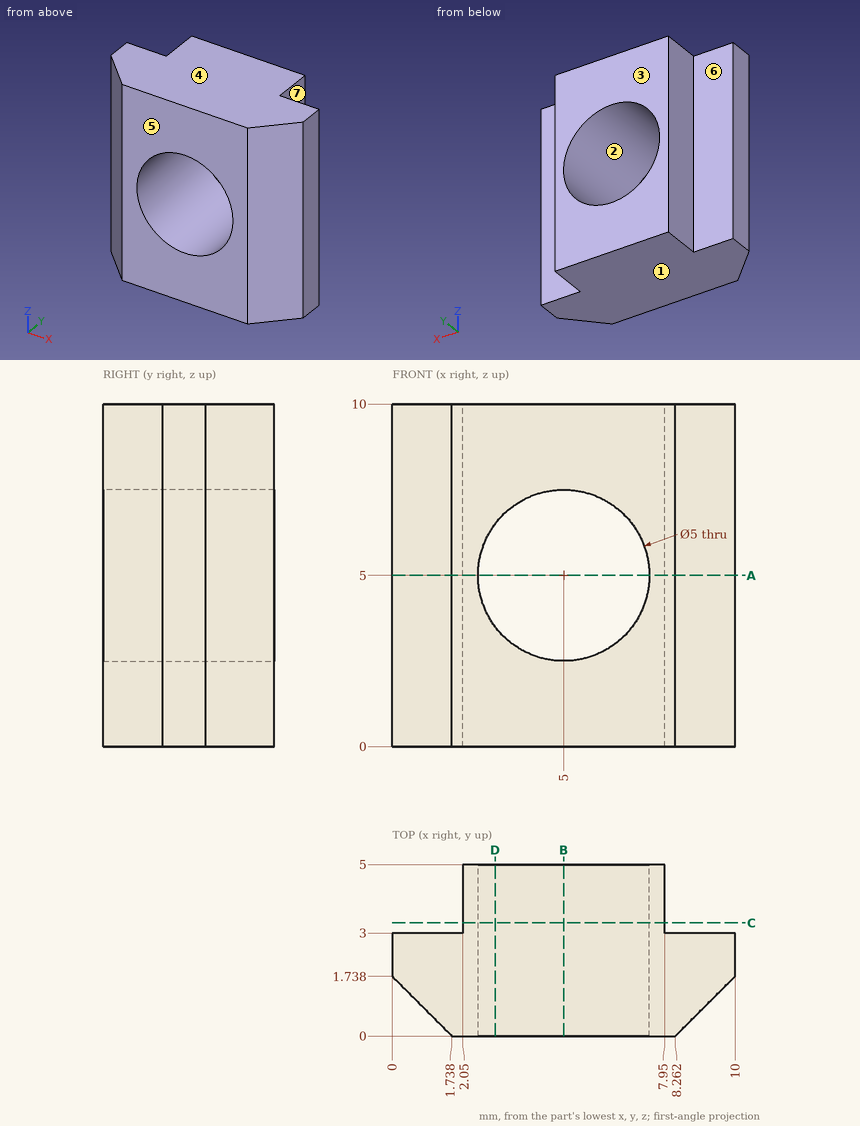
Study the drawing (mm; zero at the part's minimum x, y, z) and answer. A direction names the side the tool comes from. Round coordinates to 2 decimals unless told otherwise and drop trailing zeros. Loops run counter-clockwise (first coordinate to the right, second up) from the corner with the lowest first, then second, coordinate; pieces in that order, holes last.
Q1. Section A-A, the plane z = 5 is taken. Determine the outline of the cut face in (x, y).
Q2. Section B-B, the plane x = 5 is taken. Determine the outline of the cut face in (y, z).
Q3. Given pin 1 Ø1 at (x, z) = (9, 3) entering from +Y; pin 2 Ø1 at (y, z) = (4.5, 7) entering from +X; pin 3 Ø0.6 at (y, z) = (4, 6) entering from -X, each flat-ended and moving along its own axis, determine where each tip first touches the part or whether it passes through.
Q4. Section C-C, the plane y = 3.3 is taken. Determine the outline of the cut face in (x, z).
Q5. Find the intervals of material crossed by line 1 (X direction, y = 2.85, z = 5); line 2 (X direction, y = 4.45, z = 2); line 3 (X direction, y = 3.75, z = 5), in increasing order.
Q6. For a pull along Z with two mould halves and no side action, classify the marked faces 1, 2, 3 and 4 as released by +Z, released by -Z, zero draft, split by the parting line, or undercut.
Q7. Which of the six approach directions +Z, -Z, +X, -X, +Y, -Y give full straight-line access (tool end or side, diameter ignored) to the marked faces 5, 6 and 7?
Q8. Section D-D, the plane x = 3 is taken. Determine the outline of the cut face in (y, z).
Completed:
1. outline: (0, 1.74) - (1.74, 0) - (2.5, 0) - (2.5, 5) - (2.05, 5) - (2.05, 3) - (0, 3) - close; (7.5, 0) - (8.26, 0) - (10, 1.74) - (10, 3) - (7.95, 3) - (7.95, 5) - (7.5, 5) - close
2. outline: (0, 0) - (5, 0) - (5, 2.5) - (0, 2.5) - close; (0, 7.5) - (5, 7.5) - (5, 10) - (0, 10) - close
3. pin 1: stops at y = 3
3. pin 2: stops at x = 7.95
3. pin 3: stops at x = 2.05
4. outline: (2.05, 0) - (7.95, 0) - (7.95, 10) - (2.05, 10) - close; hole circle Ø5 at (5, 5)
5. line 1: x = 0 to 2.5, 7.5 to 10
5. line 2: x = 2.05 to 7.95
5. line 3: x = 2.05 to 2.5, 7.5 to 7.95
6. face 1: released by -Z
6. face 2: undercut
6. face 3: zero draft
6. face 4: released by +Z
7. face 5: +Z, -Z, +X, -X, -Y
7. face 6: +Z, -Z, -X, +Y
7. face 7: +Z, -Z, +X, +Y
8. outline: (0, 0) - (5, 0) - (5, 3.5) - (0, 3.5) - close; (0, 6.5) - (5, 6.5) - (5, 10) - (0, 10) - close
